Verification items for this drawing (mm, ordinates from the low corner). A direction names the side the tool comes from. Give positions to 0.01 mm unless a question says otherwise; leave off trailing zeros. Order: outer loops, then holes, each group sorted by start corner. A loop starts at its lowest first (then second) coordinate and runs counter-clockwise, first axis right, second up.
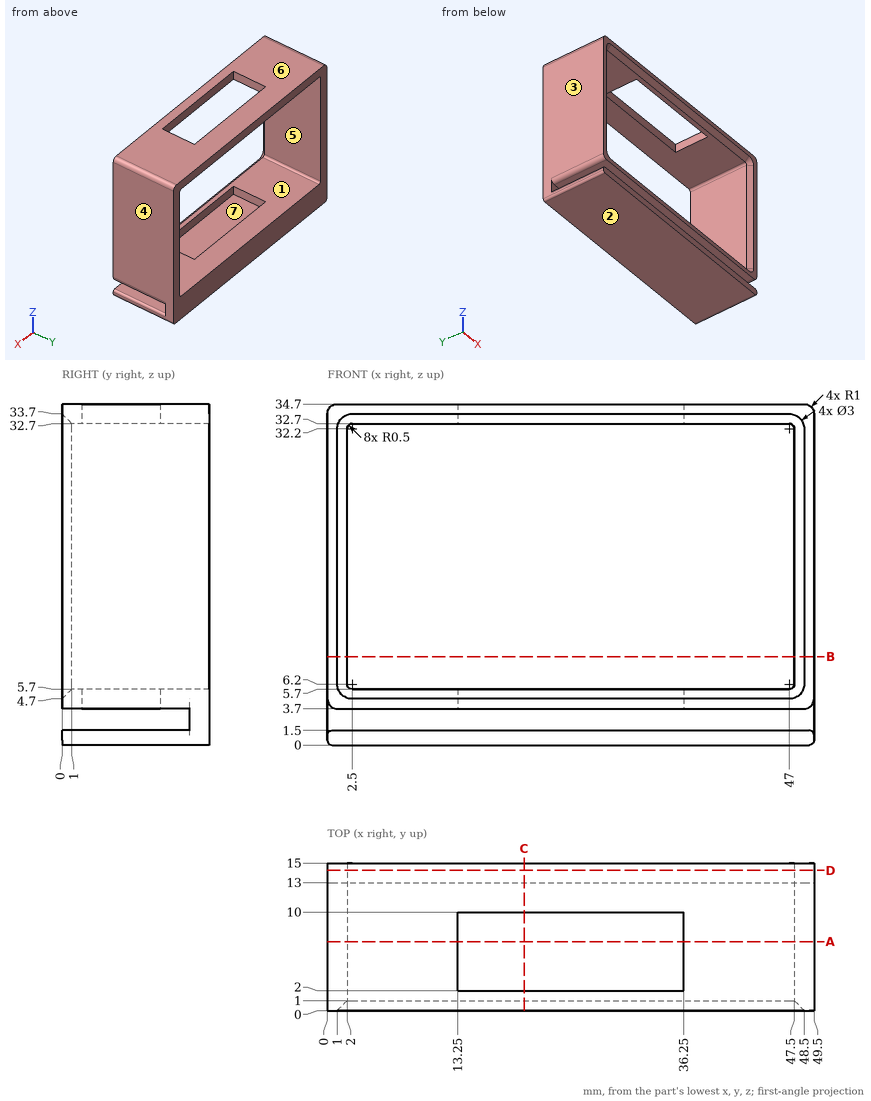
Q1. Thickness scan on L1, parallel to Z at x = 43.5, y = 4.75; L2, parallel to Z at x = 42.5, y = 13.5; L3, parallel to X at y = 2, z = 32. Record the ranges inside material, lowest first.
Q2. Release check for a two-part mould opening along X. For the marked faces 1, 2, 3 and 4 record: pulls with the +X half, pulls with the -X half, needs draft (parallel to the pull), parting line crosses it, or undercut.
Q3. Cross-section at C-C, the plane x = 20. Record the boundary of the cut face in (y, z), and give its area (3 significant figures).
Q4. Access from +Z, -Z, +X, -X, +Y, -Y to the whole of each face (thin tool, end or side, straight path). Record for the marked faces 5, 6 and 7.
Q5. Cross-section at A-A, the plane y = 7. Give the number of separate pieces and of enclosed holes in the cut face, and give its area (3 significant figures).
Q6. Gauge pin test, flat ends, axial feed: P1, Ø1, axis at y = 4, z = 4, coming from the -X side; P2, Ø10, axis at x = 35.5, z = 12.5, coming from the +Y side; P3, Ø1.1, axis at x = 34, z = 2.5, coming from the -Y side. Record the tip position at first contact, or that the pin passes through.
Q7. Cross-section at D-D, the plane y = 14.25. Record the boundary of the cut face in (x, z), and give its area (3 significant figures).
Q8. Cross-section at B-B, the plane z = 9. Record the boundary of the cut face in (x, y).
Answers follow:
1. L1: z = 0 to 1.5, 3.7 to 5.7, 32.7 to 34.7
1. L2: z = 0 to 5.7, 32.7 to 34.7
1. L3: x = 0 to 2, 47.5 to 49.5
2. face 1: undercut
2. face 2: needs draft
2. face 3: pulls with the -X half
2. face 4: pulls with the +X half
3. outline: (0, 0) - (15, 0) - (15, 5.7) - (10, 5.7) - (10, 3.7) - (13, 3.7) - (13, 1.5) - (0, 1.5) - close; (0, 3.7) - (2, 3.7) - (2, 5.7) - (1, 5.7) - (0, 4.7) - close; (0, 33.7) - (1, 32.7) - (2, 32.7) - (2, 34.7) - (0, 34.7) - close; (10, 32.7) - (15, 32.7) - (15, 34.7) - (10, 34.7) - close
3. area: 53.9 mm2
4. face 5: +Y, -Y
4. face 6: +Z, +X, -X, +Y, -Y
4. face 7: +X, -X, -Y
5. separate pieces: 3
5. enclosed holes: 0
5. area: 287 mm2
6. P1: stops at x = 0.02
6. P2: passes through
6. P3: stops at y = 13
7. outline: (0, 0.5) arc R0.5 ccw to (0.5, 0) - (49, 0) arc R0.5 ccw to (49.5, 0.5) - (49.5, 33.7) arc R1 ccw to (48.5, 34.7) - (1, 34.7) arc R1 ccw to (0, 33.7) - close; hole (2, 6.2) arc R0.5 ccw to (2.5, 5.7) - (47, 5.7) arc R0.5 ccw to (47.5, 6.2) - (47.5, 32.2) arc R0.5 ccw to (47, 32.7) - (2.5, 32.7) arc R0.5 ccw to (2, 32.2) - close
7. area: 489 mm2
8. outline: (0, 0) - (1, 0) - (2, 1) - (2, 15) - (0, 15) - close; (47.5, 1) - (48.5, 0) - (49.5, 0) - (49.5, 15) - (47.5, 15) - close
